Print and shaded views of the part. All mm, measured from the part's lowest x, y and z. Round coordinates to 2 decimals unless told otherwise and drop trailing zeros. Order: outer loops, then holes, each group sorted by start corner. A loop starts at its lowest first (then second) coordinate and runs counter-clockwise, first axis right, second up.
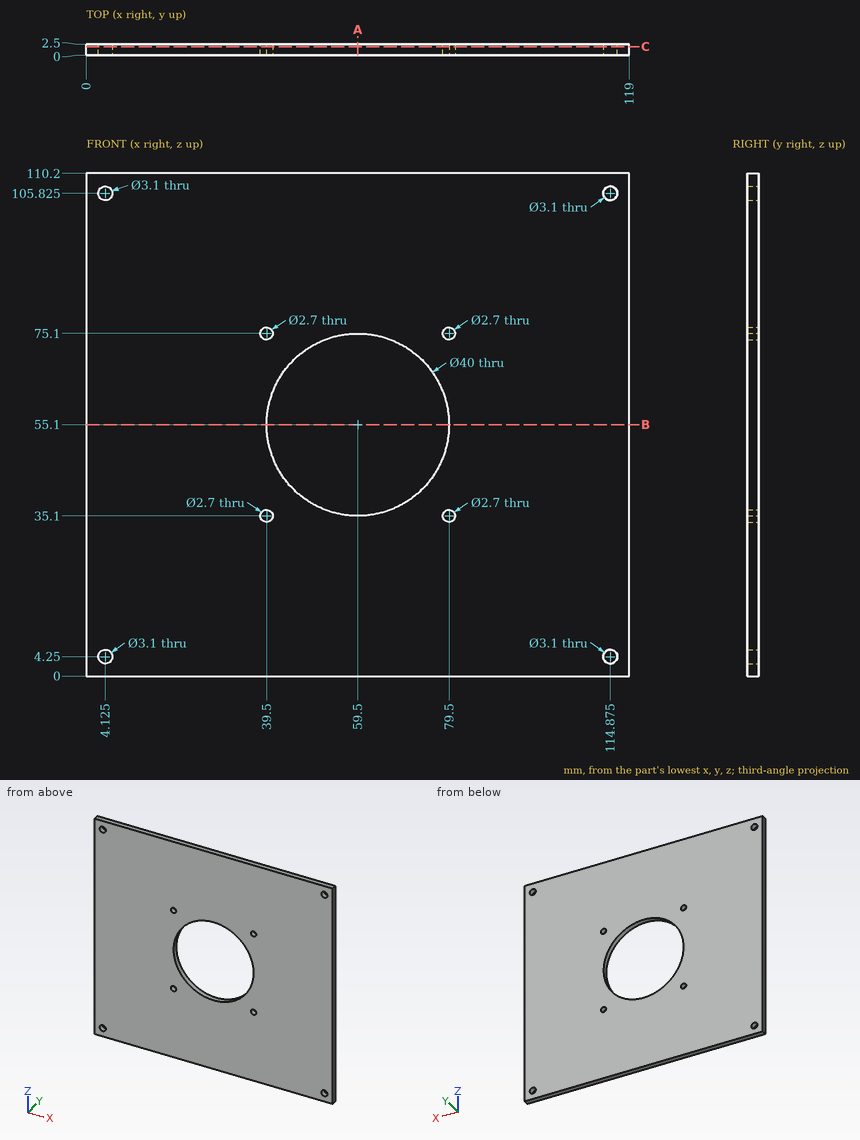
1. Pin check, flat tip, straight feed: P1, Ø1.6, axis at x = 39.5, z = 75.1, coming from the +Y side. Stop position of the tip, or through.
2. Cut at B-B, the plane z = 55.1. Write the cut outline in (x, y).
3. Cut at A-A, the plane x = 59.5. Write the cut outline in (y, z), and give its area (4 significant figures).
4. Drill centre lines: line 1 (X direction, y = 1.4, z = 4.25) (3 decimals); line 2 (Z direction, x = 114, y = 1.2); line 3 (Z direction, x = 63.5, y = 1.75). Where is each one in solid material? Low to high.
5. Cut at C-C, the plane y = 1.95. Give the number of separate pieces and of enclosed holes in the cut face, and give its area (3 significant figures).
Outcome:
1. P1: passes through
2. outline: (0, 0) - (39.5, 0) - (39.5, 2.5) - (0, 2.5) - close; (79.5, 0) - (119, 0) - (119, 2.5) - (79.5, 2.5) - close
3. outline: (0, 0) - (2.5, 0) - (2.5, 35.1) - (0, 35.1) - close; (0, 75.1) - (2.5, 75.1) - (2.5, 110.2) - (0, 110.2) - close
3. area: 175.5 mm2
4. line 1: x = 0 to 2.575, 5.675 to 113.325, 116.425 to 119
4. line 2: z = 0 to 2.97, 5.53 to 104.55, 107.1 to 110.2
4. line 3: z = 0 to 35.5, 74.7 to 110.2
5. separate pieces: 1
5. enclosed holes: 9
5. area: 11,800 mm2
